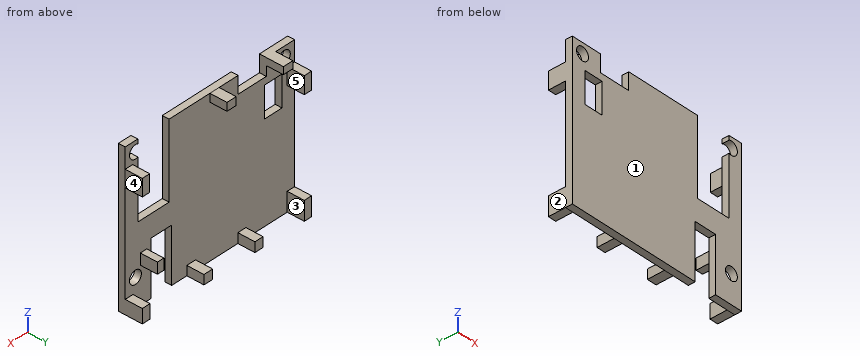
from build123d import *

# Parameters (mm, degrees)
F0_R     = 1.9
F0_W     = 5.5
F0_H     = 9
F1_DEPTH = 2
F2_W     = 2.334564
F2_H     = 5.043705
F2_H_2   = 5.546409
F2_W_2   = 2.573319
F2_H_3   = 2.870157
F2_W_3   = 2.779186
F2_H_4   = 2.767223
F2_W_4   = 2.46357
F2_H_5   = 4.105347
F2_W_5   = 2.360641
F2_H_6   = 4.940772
F2_W_6   = 2.923315
F2_H_7   = 2.368381
F2_W_7   = 3.015692
F2_H_8   = 2.129448
F2_W_8   = 2.052944
F2_H_9   = 3.241269
F3_DEPTH = 5


with BuildPart() as f1:
    # F0 (on Front) → F1 (new body)
    with BuildSketch(Plane.XZ):
        with BuildLine():
            Line((9, 0), (0, 0))
            Line((0, 0), (0, -44.5))
            Line((0, -44.5), (39.2, -44.5))
            Line((39.2, -44.5), (39.2, -28.5))
            Line((39.2, -28.5), (45.7, -28.5))
            Line((45.7, -28.5), (45.7, -44.5))
            Line((45.7, -44.5), (54, -44.5))
            Line((54, -44.5), (54, 0))
            Line((54, 0), (50, 0))
            Line((50, 0), (50, -1.254291))
            ThreePointArc((50, -1.254291), (52.65, -3), (50, -4.745709))
            Line((50, -4.745709), (50, -22))
            Line((50, -22), (40, -22))
            Line((40, -22), (40, 0))
            Line((40, 0), (18, 0))
            Line((18, 0), (18, -5))
            Line((18, -5), (9, -5))
            Line((9, -5), (9, 0))
        make_face()
        with Locations((50.75, -36.25)):
            Circle(F0_R, mode=Mode.SUBTRACT)
        with Locations((6.75, -11.5)):
            Rectangle(F0_W, F0_H, mode=Mode.SUBTRACT)
        with Locations((3.25, -3)):
            Circle(F0_R, mode=Mode.SUBTRACT)
    extrude(amount=-F1_DEPTH)

    # F2 (on face) → F3 (join)
    with BuildSketch(Plane(origin=(0, 2, 0), x_dir=(-1, 0, 0), z_dir=(0, 1, 0))):
        with Locations((-1.167282, -8.434026)):
            Rectangle(F2_W, F2_H)
        with Locations((-1.167282, -41.726795)):
            Rectangle(F2_W, F2_H_2)
        with Locations((-16.796619, -43.064921)):
            Rectangle(F2_W_2, F2_H_3)
        with Locations((-32.957062, -43.116388)):
            Rectangle(F2_W_3, F2_H_4)
        with Locations((-52.768215, -42.447327)):
            Rectangle(F2_W_4, F2_H_5)
        with Locations((-52.819679, -8.382559)):
            Rectangle(F2_W_5, F2_H_6)
        with Locations((-25.527491, -1.18419)):
            Rectangle(F2_W_6, F2_H_7)
        with Locations((-7.492154, -1.064724)):
            Rectangle(F2_W_7, F2_H_8)
        with Locations((-48.154229, -32.257447)):
            Rectangle(F2_W_8, F2_H_9)
    extrude(amount=F3_DEPTH)


solid = f1.part
Verification items for the finished model (mm, model axes). Face numbers are marked on the shaded views. A direction names the side the tool comes from. Give positions to 0.01 mm unless a question says otherwise; leave off trailing zeros. Write each loop counter-clockwise with the first axis right and the second up, starting at its lowest first coordinate (ties: lowest second). Pieces come first, ordered by that corner, then holes.
(1) Cross-section at D-D (z = -3). Enter the section's corners in (x, y).
(2) Mould release check, pull along X, two halves, no side actions. Record for the marked faces 1, 2 and 3: +X half, -X half, draft (parallel to the pull), parting line (faces both ways), or undercut.
(3) Cross-section at A-A (z = -29.5). Enter the section's corners in (x, y), plus the area to 3 significant figures.
(4) Cross-section at C-C (y = 1). Enter the section's corners in (x, z), plus the area to 3 significant figures.
(5) Access from +Z, -Z, +X, -X, +Y, -Y to the whole of each face (thin tool, end or side, straight path). Record for the marked faces 4 and 5.
(6) Cross-section at B-B (x = 50.75). Enter the section's corners in (y, z).
(7) Material ranges on line 1 (Z direction, x = 50.75, y = 0.6); line 2 (X direction, y = 1.25, z = -15); line 3 (X direction, y = 1.5, z = -5.5), recorded low to high.
(8) Gauge pin test, flat ends, axial feed: pin 1 (0.6 mm diameter, centred on x = 45.5, y = 0.5, fed in from +Z); pin 2 (1.9 mm diameter, centred on y = 4, z = -1.5, fed in from +X); pin 3 (0.8 mm diameter, centred on x = 32.5, y = 3.5, fed in from +Z). Record the tip position at first contact, or that the pin passes through.
Worked out:
1. outline: (0, 0) - (1.35, 0) - (1.35, 2) - (0, 2) - close; (5.15, 0) - (9, 0) - (9, 2) - (5.15, 2) - close; (18, 0) - (40, 0) - (40, 2) - (18, 2) - close; (52.65, 0) - (54, 0) - (54, 2) - (52.65, 2) - close
2. face 1: draft
2. face 2: -X half
2. face 3: undercut
3. outline: (0, 0) - (39.2, 0) - (39.2, 2) - (0, 2) - close; (45.7, 0) - (54, 0) - (54, 2) - (45.7, 2) - close
3. area: 95.0 mm2
4. outline: (0, -44.5) - (39.2, -44.5) - (39.2, -28.5) - (45.7, -28.5) - (45.7, -44.5) - (54, -44.5) - (54, 0) - (50, 0) - (50, -1.25) arc R1.9 cw (long way) to (50, -4.75) - (50, -22) - (40, -22) - (40, 0) - (18, 0) - (18, -5) - (9, -5) - (9, 0) - (0, 0) - close; hole circle Ø3.8 at (3.25, -3); hole (4, -16) - (9.5, -16) - (9.5, -7) - (4, -7) - close; hole circle Ø3.8 at (50.75, -36.25)
4. area: 1,950 mm2
5. face 4: +Z, -Z, +X, +Y, -Y
5. face 5: +Z, -Z, +Y
6. outline: (0, -44.5) - (2, -44.5) - (2, -38.15) - (0, -38.15) - close; (0, -34.35) - (2, -34.35) - (2, -4.9) - (0, -4.9) - close; (0, -1.1) - (2, -1.1) - (2, 0) - (0, 0) - close
7. line 1: z = -44.5 to -38.15, -34.35 to -4.9, -1.1 to 0
7. line 2: x = 0 to 4, 9.5 to 40, 50 to 54
7. line 3: x = 0 to 40, 50 to 54
8. pin 1: stops at z = -22
8. pin 2: stops at x = 26.99
8. pin 3: stops at z = -41.73
